from build123d import *

# Parameters (mm, degrees)
BOSS_EXTRUDE1_DEPTH = 76.2
CUT_EXTRUDE1_DEPTH  = 267.359355894
SKETCH4_R           = 19.05
CUT_EXTRUDE2_DEPTH  = 243.798558814


with BuildPart() as part:
    # Sketch2 → Boss-Extrude1 (new body)
    with BuildSketch(Plane.YZ):
        Polygon((0, 0), (177.8, 0), (177.8, 50.8), (21.042048969, 50.8), (-125.69533605, 197.537385018), (-161.616360534, 161.616360534), align=None)
    extrude(amount=BOSS_EXTRUDE1_DEPTH)

    # Sketch3 → Cut-Extrude1 (cut, through all)
    with BuildSketch(Plane(origin=(0, 35.921024484, 35.921024484), x_dir=(-1, 0, 0), z_dir=(0, 0.7071067811865488, 0.7071067811865464))):
        with BuildLine():
            Line((-76.2, 228.560048969), (-76.2, 152.360048969))
            ThreePointArc((-76.2, 152.360048969), (-53.881536726, 206.241585695), (0, 228.560048969))
            Line((0, 228.560048969), (-76.2, 228.560048969))
        make_face()
        with BuildLine():
            Line((0, 114.895048969), (0, 189.825048969))
            ThreePointArc((0, 189.825048969), (-37.465, 152.360048969), (0, 114.895048969))
        make_face()
        with BuildLine():
            ThreePointArc((37.465, 152.360048969), (26.491755557, 178.851804526), (0, 189.825048969))
            Line((0, 189.825048969), (0, 114.895048969))
            ThreePointArc((0, 114.895048969), (26.491755557, 125.868293411), (37.465, 152.360048969))
        make_face()
    extrude(amount=-CUT_EXTRUDE1_DEPTH, mode=Mode.SUBTRACT)

    # Sketch4 → Cut-Extrude2 (cut, through all)
    with BuildSketch(Plane.XY.offset(50.8)):
        with Locations((0, 127)):
            Circle(SKETCH4_R)
        with Locations((0, 50.8)):
            Circle(SKETCH4_R)
    extrude(amount=-CUT_EXTRUDE2_DEPTH, mode=Mode.SUBTRACT)

    # Mirror1: part across plane


with BuildPart() as part_1:
    add(part.part)
    add(part.part.mirror(Plane(origin=(0, 0, 0), x_dir=(0, 0, 1), z_dir=(1, 0, 0))))


solid = part_1.part
Read the model definition and answer for the solid it produces. Units are mm, in the model's axes. Round coordinates to 2 decimals unless told otherwise and drop trailing zeros. Write each loop counter-clockwise with the first axis right and the second up, starting at its lowest first coordinate (ties: lowest second). Pieces come first, ordered by that corner, then holes. Notation, with made-up numbers: M -14,-4.75 L 15,-4.75 A13 cw 15,0.25 Z; hole C 75.25,71 d6. An arc over 180 degrees is marked long. Use a Markdown table: item, result.
1) The part is cut by section A-A (y = 127). Write down the section's boundary in (x, z).
Answers follow:
| item | result |
|---|---|
| outline | M -76.2,0 L -19.05,0 L -19.05,50.8 L -76.2,50.8 Z; M 19.05,0 L 76.2,0 L 76.2,50.8 L 19.05,50.8 Z |
2) For a pull along Z with two mould halves and no side action, classify faces 1 (the flat face through (1, 101, 50.8)), 2 (the cylindrical face through (36.574, -83.78, 120.204)), 3 (the flat face through (1, -64, 64)), 4 (the flat face through (1, 177.8, 25)) as pulls with the +Z half, pulls with the -Z half, needs draft (parallel to the pull), parting line crosses it, or undercut.
Answers follow:
| item | result |
|---|---|
| face 1 | pulls with the +Z half |
| face 2 | undercut |
| face 3 | pulls with the -Z half |
| face 4 | needs draft |
3) The part is cut by section C-C (x = 11). Write down the section's boundary in (y, z).
Answers follow:
| item | result |
|---|---|
| outline | M -161.05,161.05 L -133.06,133.06 L -97.14,168.98 L -125.13,196.97 Z; M -82.41,82.41 L 0,0 L 35.25,0 L 35.25,50.8 L 21.04,50.8 L -46.49,118.33 Z; M 66.35,0 L 111.45,0 L 111.45,50.8 L 66.35,50.8 Z; M 142.55,0 L 177.8,0 L 177.8,50.8 L 142.55,50.8 Z |
4) The part is cut by section D-D (y = 77). Write down the section's boundary in (x, z).
Answers follow:
| item | result |
|---|---|
| outline | M -76.2,0 L 76.2,0 L 76.2,50.8 L -76.2,50.8 Z |
5) Flat-ended cylindrical pins translate along their axes: pin 1 (1.5 mm diameter, centred on x = 13.5, z = 99.5, fed in from -Y); pin 2 (12 mm diameter, centred on x = -11.5, z = 108, fed in from +Y); pin 3 (1 mm diameter, centred on x = -56.5, y = 26, fed in from -Z); pin 4 (12 mm diameter, centred on x = 54, y = -78, fed in from +Z). Find the tip coordinate at first contact, or state that the pin passes through.
Answers follow:
| item | result |
|---|---|
| pin 1 | stops at y = -67.4 |
| pin 2 | stops at y = -30.16 |
| pin 3 | stops at z = 0 |
| pin 4 | stops at z = 155.84 |
6) Straight lines are drawn through the part: line 1 along X through (y, z) = (127, 30); line 2 along Y through (x, z) = (13, 10); line 3 along Y through (x, z) = (0, 31). For each, find the intervals that lie inside material, in ascending order. Write a range as [from, to].
Answers follow:
| item | result |
|---|---|
| line 1 | x = [-76.2, -19.05], [19.05, 76.2] |
| line 2 | y = [-10, 36.88], [64.72, 113.08], [140.92, 177.8] |
| line 3 | y = [-31, 31.75], [69.85, 107.95], [146.05, 177.8] |
7) The part is cut by section B-B (z = 39). Write down the section's boundary in (x, y).
Answers follow:
| item | result |
|---|---|
| outline | M -76.2,-39 L 76.2,-39 L 76.2,177.8 L -76.2,177.8 Z; hole C 0,50.8 d38.1; hole C 0,127 d38.1 |
